Could you check a few things on this model? Use its own coordinates, in mm. Face numbers are marked on the shaded views. A direction names the side the tool comes from. Coordinates: 2 decimals unless noted, no trailing zeros. Order: outer loops, then holes, each group sorted by start corner. A loop starts at its lowest first (then second) coordinate and runs counter-clockwise, first axis right, second up. Notation, with made-up numbers: (45, -2) -> (54, -2) arc R32 ccw to (54, 31) -> close; hole circle Ø2 at (14.25, 70.5). An arc over 180 degrees is marked (long way). Put each result on its own line as item: value. Start each with the question number.
Q1. If we section it at A-A (z = -337.5): Please give me the cut outline in (x, y).
Q2. Please list where these lines run through material, in increasing order: line 1 along Z through (x, y) = (568, 65.5); line 2 along X through (y, z) = (83, -253); line 3 along X through (y, z) = (23.5, 204).
Q3. We'd pull the mould along Z, two halves only. Please class the marked faces 1 and 2: +Z half, -Z half, draft (parallel to the pull), parting line (faces both ways), or undercut.
Q4. If we section it at B-B (x = -1): Please give me the cut outline in (y, z).
Q5. For the marked faces 3 and 4, which set-ups out of +Z, -Z, +X, -X, +Y, -Y let a thin tool reach every point of the face, with its end or its side?
Q6. If we section it at C-C (y = 79.5): Please give me the cut outline in (x, z), and give its area (3 significant figures).
Q7. Will these pins go through, and if not, where does the flat tip stop? pin 1 (5 mm diameter, centred on y = 105, z = -199.5, fed in from -X); pin 2 (5 mm diameter, centred on x = 371.5, y = 13, fed in from +Z).
from build123d import *

# Parameters (mm, degrees)
SKETCH1_W           = 998.22
SKETCH1_H           = 863.6
BOSS_EXTRUDE1_DEPTH = 127
SKETCH2_W           = 820.42
SKETCH2_H           = 685.8
CUT_EXTRUDE1_DEPTH  = 127
FILLET1_R           = 25.4


with BuildPart() as part:
    # Sketch1 → Boss-Extrude1 (new body)
    with BuildSketch(Plane(origin=(0, 0, 0), x_dir=(1, 0, 0), z_dir=(0, 1, 0))):
        with Locations((226.123239937, 18.056640537)):
            Rectangle(SKETCH1_W, SKETCH1_H)
    extrude(amount=BOSS_EXTRUDE1_DEPTH)

    # Sketch2 → Cut-Extrude1 (cut)
    with BuildSketch(Plane.XZ):
        with Locations((226.123239937, -18.056640537)):
            Rectangle(SKETCH2_W, SKETCH2_H)
    extrude(amount=-CUT_EXTRUDE1_DEPTH, mode=Mode.SUBTRACT)

    # Fillet1
    fillet1_edges = [part.edges().sort_by_distance(p)[0] for p in [
        (-272.986760063, 63.5, 413.743359463),
        (-272.986760063, 63.5, -449.856640537),
        (-272.986760063, 0, -18.056640537),
        (-272.986760063, 127, -18.056640537),
        (725.233239937, 63.5, 413.743359463),
        (226.123239937, 0, 413.743359463),
        (226.123239937, 127, 413.743359463),
        (725.233239937, 63.5, -449.856640537),
        (226.123239937, 0, -449.856640537),
        (226.123239937, 127, -449.856640537),
        (725.233239937, 0, -18.056640537),
        (725.233239937, 127, -18.056640537),
    ]]
    fillet(fillet1_edges, radius=FILLET1_R)


solid = part.part
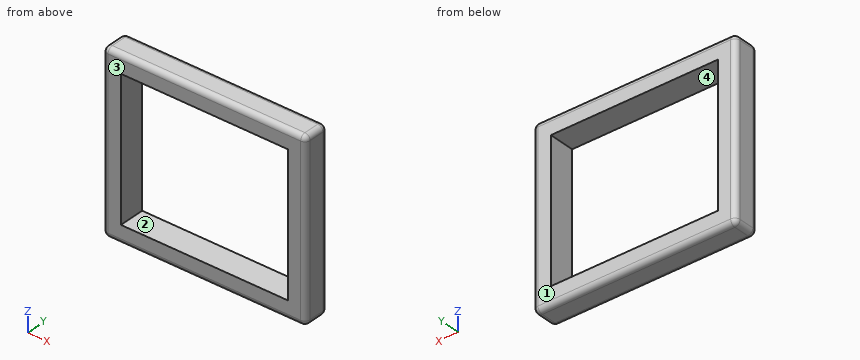
The answers:
1. outline: (-272.99, 25.4) arc R25.4 ccw to (-247.59, 0) -> (-184.09, 0) -> (-184.09, 127) -> (-247.59, 127) arc R25.4 ccw to (-272.99, 101.6) -> close; (636.33, 0) -> (699.83, 0) arc R25.4 ccw to (725.23, 25.4) -> (725.23, 101.6) arc R25.4 ccw to (699.83, 127) -> (636.33, 127) -> close
2. line 1: -449.86 to -360.96, 324.84 to 413.74
2. line 2: -272.99 to -184.09, 636.33 to 725.23
2. line 3: -272.92 to -184.09, 636.33 to 725.16
3. face 1: draft
3. face 2: undercut
4. outline: (0, -424.46) arc R25.4 ccw to (25.4, -449.86) -> (101.6, -449.86) arc R25.4 ccw to (127, -424.46) -> (127, -360.96) -> (0, -360.96) -> close; (0, 324.84) -> (127, 324.84) -> (127, 388.34) arc R25.4 ccw to (101.6, 413.74) -> (25.4, 413.74) arc R25.4 ccw to (0, 388.34) -> close
5. face 3: +Z, -Z, +X, -X, -Y
5. face 4: +Y, -Y
6. outline: (-272.99, -424.46) arc R25.4 ccw to (-247.59, -449.86) -> (699.83, -449.86) arc R25.4 ccw to (725.23, -424.46) -> (725.23, 388.34) arc R25.4 ccw to (699.83, 413.74) -> (-247.59, 413.74) arc R25.4 ccw to (-272.99, 388.34) -> close; hole (-184.09, -360.96) -> (636.33, -360.96) -> (636.33, 324.84) -> (-184.09, 324.84) -> close
6. area: 299,000 mm^2
7. pin 1: x = -272.97
7. pin 2: z = 411.73
